Autodesk Inventor part; units mm, degrees
ref_plane "Work Plane1" through (0, 0, -21.5) normal (0, 0, 1) x (1, 0, 0)
ref_plane "Work Plane2" through (0, 0, -2) normal (0, 0, 1) x (1, 0, 0)
ref_plane "YZ Plane" through (0, 0, 0) normal (1, 0, 0) x (0, 1, 0)
sketch "Sketch2" plane through (0, 0, 0) normal (0, 0, 1) x (1, 0, 0)
  circle A0 centre (0, 0) radius 1.9
  dimension "d0" = 3.8
extrude "Extrusion1" add sketch "Sketch2" against normal blind 12.5
fillet "Fillet1" radius 1.9 1 edges at (-1.9, 0, -12.5)
sketch "Sketch3" plane through (0, 0, 0) normal (0, 1, 0) x (-1, 0, 0)
  line L0 (1.9, 0) -> (-1.9, 0) construction
  arc A0 (-3.4256, -17.2823) -> (3.4256, -17.2823) centre (0, -18) ccw
  line L1 (3.4256, -17.2823) -> (1.9, -10)
  line L2 (-3.4256, -17.2823) -> (-1.9, -10)
  line L3 (0, -27.6) -> (0, 4.6) construction
  line L4 (1.9, 0) -> (1.9, -10.6) construction
  line L5 (-1.9, 0) -> (-1.9, -10.6) construction
  line L6 (-1.9, -10) -> (1.9, -10)
  point P0 (0, 0)
  point P1 (-2.75, -11.75)
  point P2 (2.75, -11.75)
  dimension "d4" = 7
  dimension "d5" = 10
  dimension "d6" = 18
  dimension "d7" = 10
extrude "Extrusion2" add sketch "Sketch3" along normal mid plane 2.5
sketch "Sketch4" plane through (0, 0, 0) normal (0, 1, 0) x (-1, 0, 0)
  arc A0 (-3.4256, -17.2823) -> (3.4256, -17.2823) centre (0, -18) ccw construction
  arc A1 (-2.4, -18) -> (2.4, -18) centre (0, -18) ccw
  line L0 (2.4, -18) -> (-2.4, -18)
  point P0 (0, 0)
  dimension "d10" = 4.8
revolve "Revolution1" cut sketch "Sketch4" angle 360 about axis through (-2.4, 0, -18) along (1, 0, 0)
sketch "Sketch5" plane through (0, 0, 0) normal (0, 0, 1) x (1, 0, 0)
  circle A0 centre (0, 0) radius 1
  dimension "d12" = 2
extrude "Extrusion3" cut sketch "Sketch5" against normal blind 12
thread "Thread1"
ref_plane "Work Plane1" through (0, 0, -21.5) normal (0, 0, 1) x (1, 0, 0)
sketch "Sketch6" plane through (0, 0, -21.5) normal (0, 0, 1) x (1, 0, 0)
  line L0 (-4.9, 0) -> (4.9, 0) construction
  line L1 (0, -2.66) -> (0, 2.66) construction
  line L2 (1.9, 0.7) -> (-1.9, 0.7)
  line L3 (-1.9, 0.7) -> (-1.9, -0.7)
  line L4 (-1.9, -0.7) -> (1.9, -0.7)
  line L5 (1.9, -0.7) -> (1.9, 0.7)
  point P0 (0, 0)
  dimension "d17" = 3.8
  dimension "d18" = 1.4
extrude "Extrusion4" add sketch "Sketch6" against normal blind 1
sketch "Sketch7" plane through (0, 0, -21.5) normal (0, 0, 1) x (1, 0, 0)
  line L0 (-1.9, -0.7) -> (-1.9, 0.7) construction
  line L1 (-1.9, 0.7) -> (1.9, 0.7) construction
  line L2 (1.9, 0.7) -> (1.9, -0.7) construction
  line L3 (1.9, -0.7) -> (-1.9, -0.7) construction
  line L4 (-1.9, 0.7) -> (1.9, 0.7)
  line L5 (1.9, 0.7) -> (1.9, -0.7)
  line L6 (1.9, -0.7) -> (-1.9, -0.7)
  line L7 (-1.9, -0.7) -> (-1.9, 0.7)
  point P0 (0, 0)
extrude "Extrusion5" add sketch "Sketch7" along normal up to surface
ref_plane "Work Plane2" through (0, 0, -2) normal (0, 0, 1) x (1, 0, 0)
sketch "Sketch8" plane through (0, 0, -2) normal (0, 0, 1) x (1, 0, 0)
  arc A0 (1.4309, 1.25) -> (-1.4309, 1.25) centre (0, 0) ccw construction
  circle A1 centre (0, 0) radius 1.9
  line L0 (0, -2.98) -> (0, 4.58) construction
  line L1 (-2.66, 0) -> (2.66, 0) construction
  line L2 (-1, 1.6155) -> (0, 2.9)
  line L3 (1, 1.6155) -> (0, 2.9)
  dimension "d24" = 2.9
  dimension "d25" = 2
extrude "Extrusion6" add sketch "Sketch8" against normal blind 8 contours A1 L2 L3
mirror "Mirror1" about plane through (0, 0, 0) normal (0, 1, 0) of "Extrusion6"
equation "\"d5\" = d7"
properties part number "Rotule_M2" material "POM"
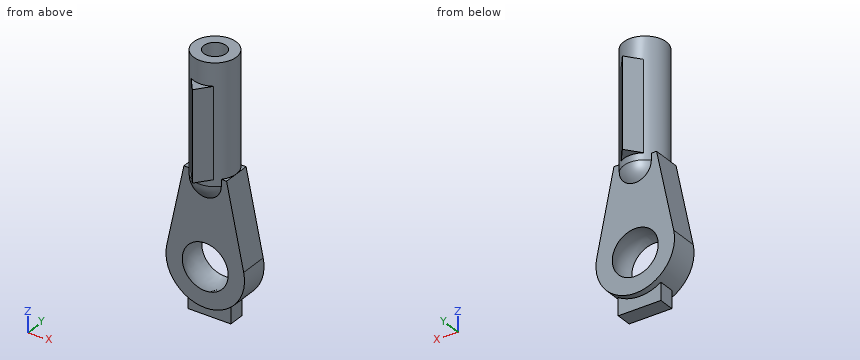
Design review of the part built by this model. Coordinates are the model's own, in mm. Give positions to 0.01 mm unless a question says otherwise; leave off trailing zeros. Order: outer loops, then holes, each group sorted by start corner. A loop starts at its lowest first (then second) coordinate and runs counter-clockwise, first axis right, second up. Notation, with made-up numbers: (-11, 15) -> (25, 15) arc R19 cw to (25, 20) -> close; hole circle Ø4 at (2.5, 32.25). An arc over 180 degrees is marked (long way). Write each question's results on one line, items separated by ' | '. Start each with the question number.
Q1. Add section C-C on z = -18. Give the boundary of the cut face in (x, y).
Q2. Add section B-B on x = -0.75. Give the boundary of the cut face in (y, z).
Q3. For pin 1 (1 mm diameter, centred on x = 0, y = -2.5, fed in from +Z); pin 2 (0.6 mm diameter, centred on x = 0, y = -2.5, fed in from -Z); pin 3 (1 mm diameter, centred on y = 1.5, z = -19, fed in from -X), all flat-tipped, find the tip position at first contact; note any pin that passes through.
Q4. Add section A-A on z = -8. Give the boundary of the cut face in (x, y).
Q5. Wall thickness on L1, parallel to Z at x = 0.25, y = -0.1; L2, parallel to X at y = -0.9, z = -6; L3, parallel to Z at x = -1.5, y = -0.95: over which ranges is each line inside the solid? List them lowest first. Write a range as from..to.
Q6. Add section D-D on z = -11.5. Give the boundary of the cut face in (x, y), and give its area (3 significant figures).
Found:
1) outline: (-3.5, -1.25) -> (-2.05, -1.25) arc R2.4 cw to (-2.05, 1.25) -> (-3.5, 1.25) -> close; (2.05, -1.25) -> (3.5, -1.25) -> (3.5, 1.25) -> (2.05, 1.25) arc R2.4 cw to start
2) outline: (-1.94, -10) -> (-1.75, -10) -> (-1.75, -10.6) arc R1.75 ccw to (-1.25, -11.82) -> (-1.25, -16.09) arc R2.28 cw to (1.25, -16.09) -> (1.25, -11.82) arc R1.75 ccw to (1.75, -10.6) -> (1.75, -10) -> (1.94, -10) -> (1.94, -2) -> (1.75, -2) -> (1.75, 0) -> (0.66, 0) -> (0.66, -12) -> (-0.66, -12) -> (-0.66, 0) -> (-1.75, 0) -> (-1.75, -2) -> (-1.94, -2) -> close; (-1.25, -21.42) -> (-0.7, -21.42) -> (-0.7, -22.5) -> (0.7, -22.5) -> (0.7, -21.42) -> (1.25, -21.42) -> (1.25, -19.91) arc R2.28 cw to (-1.25, -19.91) -> close
3) pin 1: stops at z = -2 | pin 2: stops at z = -10 | pin 3: stops at x = -3.45
4) outline: (-1, -1.62) -> (0, -2.9) -> (1, -1.62) arc R1.9 ccw to (1, 1.62) -> (0, 2.9) -> (-1, 1.62) arc R1.9 ccw to start; hole circle Ø2 at (0, 0)
5) L1: z = -22.5..-20.38, -15.62..-12 | L2: x = -1.67..-0.44, 0.44..1.67 | L3: z = -21.16..-19.61, -16.39..0
6) outline: (-2.21, -1.25) -> (-1.11, -1.25) arc R1.67 ccw to (1.11, -1.25) -> (2.21, -1.25) -> (2.21, 1.25) -> (1.11, 1.25) arc R1.67 ccw to (-1.11, 1.25) -> (-2.21, 1.25) -> close; hole circle Ø2 at (0, 0) | area: 9.22 mm2
